```python
from build123d import *

# Parameters (mm, degrees)
SKETCH1_R           = 1.5
BOSS_EXTRUDE1_DEPTH = 5


with BuildPart() as part:
    # Sketch1 → Boss-Extrude1 (new body)
    with BuildSketch(Plane.XY):
        with BuildLine():
            Line((-15, 92), (-10, 97))
            Line((-10, 97), (-5, 97))
            ThreePointArc((-5, 97), (-1.464466094, 98.464466094), (0, 102))
            Line((0, 102), (0, 107))
            ThreePointArc((0, 107), (0.878679656, 109.121320344), (3, 110))
            Line((3, 110), (14.566367929, 110))
            ThreePointArc((14.566367929, 110), (18.101901835, 111.464466094), (19.566367929, 115))
            Line((19.566367929, 115), (19.566367929, 142))
            Line((19.566367929, 142), (22.566367929, 145))
            Line((22.566367929, 145), (86.566367929, 145))
            Line((86.566367929, 145), (89.566367929, 142))
            Line((89.566367929, 142), (89.566367929, 115))
            ThreePointArc((89.566367929, 115), (91.030834023, 111.464466094), (94.566367929, 110))
            Line((94.566367929, 110), (106.132735857, 110))
            ThreePointArc((106.132735857, 110), (108.254056201, 109.121320344), (109.132735857, 107))
            Line((109.132735857, 107), (109.132735857, 102))
            ThreePointArc((109.132735857, 102), (110.597201951, 98.464466094), (114.132735857, 97))
            Line((114.132735857, 97), (119.132735857, 97))
            Line((119.132735857, 97), (124.132735857, 92))
            Line((124.132735857, 92), (124.132735857, 18))
            Line((124.132735857, 18), (119.132735857, 13))
            Line((119.132735857, 13), (114.132735857, 13))
            ThreePointArc((114.132735857, 13), (110.597201951, 11.535533906), (109.132735857, 8))
            Line((109.132735857, 8), (109.132735857, 3))
            ThreePointArc((109.132735857, 3), (108.254056201, 0.878679656), (106.132735857, 0))
            Line((106.132735857, 0), (94.566367929, 0))
            ThreePointArc((94.566367929, 0), (91.030834023, -1.464466094), (89.566367929, -5))
            Line((89.566367929, -5), (89.566367929, -32))
            Line((89.566367929, -32), (86.566367929, -35))
            Line((86.566367929, -35), (22.566367929, -35))
            Line((22.566367929, -35), (19.566367929, -32))
            Line((19.566367929, -32), (19.566367929, -5))
            ThreePointArc((19.566367929, -5), (18.101901835, -1.464466094), (14.566367929, 0))
            Line((14.566367929, 0), (3, 0))
            ThreePointArc((3, 0), (0.878679656, 0.878679656), (0, 3))
            Line((0, 3), (0, 9.1034271))
            ThreePointArc((0, 9.1034271), (-1.464466094, 12.638961006), (-5, 14.1034271))
            Line((-5, 14.1034271), (-10, 14.1034271))
            Line((-10, 14.1034271), (-15, 19.1034271))
            Line((-15, 19.1034271), (-15, 92))
        make_face()
        with Locations((54.566367929, 97)):
            Circle(SKETCH1_R, mode=Mode.SUBTRACT)
        with Locations((54.566367929, 13)):
            Circle(SKETCH1_R, mode=Mode.SUBTRACT)
        with Locations((96.132735857, 55)):
            Circle(SKETCH1_R, mode=Mode.SUBTRACT)
        with Locations((13, 55)):
            Circle(SKETCH1_R, mode=Mode.SUBTRACT)
        with BuildLine():
            Line((34.566367929, 133), (74.566367929, 133))
            ThreePointArc((74.566367929, 133), (76.687688272, 132.121320344), (77.566367929, 130))
            Line((77.566367929, 130), (77.566367929, 118))
            ThreePointArc((77.566367929, 118), (76.687688272, 115.878679656), (74.566367929, 115))
            Line((74.566367929, 115), (34.566367929, 115))
            ThreePointArc((34.566367929, 115), (32.445047585, 115.878679656), (31.566367929, 118))
            Line((31.566367929, 118), (31.566367929, 130))
            ThreePointArc((31.566367929, 130), (32.445047585, 132.121320344), (34.566367929, 133))
        make_face(mode=Mode.SUBTRACT)
        with BuildLine():
            Line((34.566367929, -23), (74.566367929, -23))
            ThreePointArc((74.566367929, -23), (76.687688272, -22.121320344), (77.566367929, -20))
            Line((77.566367929, -20), (77.566367929, -8))
            ThreePointArc((77.566367929, -8), (76.687688272, -5.878679656), (74.566367929, -5))
            Line((74.566367929, -5), (34.566367929, -5))
            ThreePointArc((34.566367929, -5), (32.445047585, -5.878679656), (31.566367929, -8))
            Line((31.566367929, -8), (31.566367929, -20))
            ThreePointArc((31.566367929, -20), (32.445047585, -22.121320344), (34.566367929, -23))
        make_face(mode=Mode.SUBTRACT)
        with BuildLine():
            Line((-7.610040083, 24.1034271), (-7.610040083, 87))
            ThreePointArc((-7.610040083, 87), (-5, 89.610040083), (-2.389959917, 87))
            Line((-2.389959917, 87), (-2.389959917, 24.1034271))
            ThreePointArc((-2.389959917, 24.1034271), (-5, 21.493387017), (-7.610040083, 24.1034271))
        make_face(mode=Mode.SUBTRACT)
        with BuildLine():
            Line((116.74277594, 24.1034271), (116.74277594, 87))
            ThreePointArc((116.74277594, 87), (114.132735857, 89.610040083), (111.522695774, 87))
            Line((111.522695774, 87), (111.522695774, 24.1034271))
            ThreePointArc((111.522695774, 24.1034271), (114.132735857, 21.493387017), (116.74277594, 24.1034271))
        make_face(mode=Mode.SUBTRACT)
        with BuildLine():
            Line((21.529947274, 89.468147489), (88.351003471, 25.308726653))
            ThreePointArc((88.351003471, 25.308726653), (88.386999729, 23.537331865), (86.615604941, 23.501335607))
            Line((86.615604941, 23.501335607), (19.794548743, 87.660756443))
            ThreePointArc((19.794548743, 87.660756443), (19.758552485, 89.432151231), (21.529947274, 89.468147489))
        make_face(mode=Mode.SUBTRACT)
        with BuildLine():
            Line((30.141972391, 90.830211564), (90.687510201, 32.696340879))
            ThreePointArc((90.687510201, 32.696340879), (90.727054178, 30.750360947), (88.781074246, 30.71081697))
            Line((88.781074246, 30.71081697), (28.235536436, 88.844687655))
            ThreePointArc((28.235536436, 88.844687655), (28.195992459, 90.790667587), (30.141972391, 90.830211564))
        make_face(mode=Mode.SUBTRACT)
        with BuildLine():
            Line((39.483266545, 90.686865308), (90.503044374, 41.699321816))
            ThreePointArc((90.503044374, 41.699321816), (90.542042113, 39.780222555), (88.622942851, 39.741224816))
            Line((88.622942851, 39.741224816), (37.603165023, 88.728768307))
            ThreePointArc((37.603165023, 88.728768307), (37.564167284, 90.647867569), (39.483266545, 90.686865308))
        make_face(mode=Mode.SUBTRACT)
        with BuildLine():
            Line((49.153982666, 90.837738164), (90.341625616, 51.290693151))
            ThreePointArc((90.341625616, 51.290693151), (90.381469395, 49.329959822), (88.420736066, 49.290116043))
            Line((88.420736066, 49.290116043), (47.233093116, 88.837161056))
            ThreePointArc((47.233093116, 88.837161056), (47.193249337, 90.797894385), (49.153982666, 90.837738164))
        make_face(mode=Mode.SUBTRACT)
        with BuildLine():
            Line((58.913272098, 90.890808974), (90.212200397, 60.838588511))
            ThreePointArc((90.212200397, 60.838588511), (90.254158107, 58.773827493), (88.189397089, 58.731869782))
            Line((88.189397089, 58.731869782), (56.89046879, 88.784090246))
            ThreePointArc((56.89046879, 88.784090246), (56.84851108, 90.848851264), (58.913272098, 90.890808974))
        make_face(mode=Mode.SUBTRACT)
        with BuildLine():
            Line((68.200844973, 90.997320319), (90.14380499, 69.928398542))
            ThreePointArc((90.14380499, 69.928398542), (90.190005291, 67.654857424), (87.916464173, 67.608657123))
            Line((87.916464173, 67.608657123), (65.973504156, 88.677578901))
            ThreePointArc((65.973504156, 88.677578901), (65.927303856, 90.951120018), (68.200844973, 90.997320319))
        make_face(mode=Mode.SUBTRACT)
        with BuildLine():
            Line((75.985646215, 90.418887754), (89.801777498, 77.153084552))
            ThreePointArc((89.801777498, 77.153084552), (89.839647655, 75.289474178), (87.976037281, 75.251604021))
            Line((87.976037281, 75.251604021), (74.159905999, 88.517407223))
            ThreePointArc((74.159905999, 88.517407223), (74.122035842, 90.381017597), (75.985646215, 90.418887754))
        make_face(mode=Mode.SUBTRACT)
        with BuildLine():
            Line((84.164714184, 90.316514556), (89.552781085, 85.143066673))
            ThreePointArc((89.552781085, 85.143066673), (89.586573484, 83.480124936), (87.923631748, 83.446332537))
            Line((87.923631748, 83.446332537), (82.535564847, 88.619780421))
            ThreePointArc((82.535564847, 88.619780421), (82.501772448, 90.282722157), (84.164714184, 90.316514556))
        make_face(mode=Mode.SUBTRACT)
        with BuildLine():
            Line((20.116699843, 25.040162824), (25.391558074, 19.751335111))
            ThreePointArc((25.391558074, 19.751335111), (27.054841666, 19.749135575), (27.057041202, 21.412419167))
            Line((27.057041202, 21.412419167), (21.782182971, 26.701246879))
            ThreePointArc((21.782182971, 26.701246879), (20.118899379, 26.703446416), (20.116699843, 25.040162824))
        make_face(mode=Mode.SUBTRACT)
        with BuildLine():
            Line((19.858987713, 33.215810662), (33.384828271, 19.654149429))
            ThreePointArc((33.384828271, 19.654149429), (35.248821752, 19.651684473), (35.251286708, 21.515677954))
            Line((35.251286708, 21.515677954), (21.72544615, 35.077339187))
            ThreePointArc((21.72544615, 35.077339187), (19.861452669, 35.079804143), (19.858987713, 33.215810662))
        make_face(mode=Mode.SUBTRACT)
        with BuildLine():
            Line((19.132791007, 40.988220389), (40.614707507, 19.449413025))
            ThreePointArc((40.614707507, 19.449413025), (42.888716002, 19.446405862), (42.891723164, 21.720414358))
            Line((42.891723164, 21.720414358), (21.409806664, 43.259221722))
            ThreePointArc((21.409806664, 43.259221722), (19.135798169, 43.262228884), (19.132791007, 40.988220389))
        make_face(mode=Mode.SUBTRACT)
        with BuildLine():
            Line((19.062870224, 50.276140805), (49.704176763, 19.55368646))
            ThreePointArc((49.704176763, 19.55368646), (51.76936224, 19.550955446), (51.772093254, 21.616140923))
            Line((51.772093254, 21.616140923), (21.130786715, 52.338595268))
            ThreePointArc((21.130786715, 52.338595268), (19.065601238, 52.341326282), (19.062870224, 50.276140805))
        make_face(mode=Mode.SUBTRACT)
        with BuildLine():
            Line((18.930558524, 60.034677598), (59.252807938, 19.6056422))
            ThreePointArc((59.252807938, 19.6056422), (61.21394434, 19.603048781), (61.216537759, 21.564185183))
            Line((61.216537759, 21.564185183), (20.894288344, 61.993220582))
            ThreePointArc((20.894288344, 61.993220582), (18.933151942, 61.995814), (18.930558524, 60.034677598))
        make_face(mode=Mode.SUBTRACT)
        with BuildLine():
            Line((18.897713631, 69.706514762), (68.845514944, 19.626435978))
            ThreePointArc((68.845514944, 19.626435978), (70.76500872, 19.623897628), (70.76754707, 21.543391404))
            Line((70.76754707, 21.543391404), (20.819745757, 71.623470187))
            ThreePointArc((20.819745757, 71.623470187), (18.900251981, 71.626008538), (18.897713631, 69.706514762))
        make_face(mode=Mode.SUBTRACT)
        with BuildLine():
            Line((18.576959915, 79.043400842), (77.850375474, 19.613010658))
            ThreePointArc((77.850375474, 19.613010658), (79.796755446, 19.610436753), (79.79932935, 21.556816725))
            Line((79.79932935, 21.556816725), (20.525913792, 80.98720691))
            ThreePointArc((20.525913792, 80.98720691), (18.57953382, 80.989780815), (18.576959915, 79.043400842))
        make_face(mode=Mode.SUBTRACT)
    extrude(amount=BOSS_EXTRUDE1_DEPTH)


solid = part.part
```
Work out the finished part from the listing and answer in its coordinate system (mm). A direction names the side the tool comes from. Coordinates: 2 decimals unless noted, no trailing zeros. Answer as a JSON object with one key per item and string values.
Q1. Given pin 1 Ø2.5 at (y, z) = (130, 1.5) entering from +X; pin 2 Ø1.5 at (x, z) = (17.5, 2.5) entering from +Y; pin 3 Ø2.5 at (y, z) = (-13.5, 2.5) entering from -X, each flat-ended and moving along its own axis, determine where each tip first touches the part or whether it passes through.
Results list:
{"pin 1": "stops at x = 89.57", "pin 2": "stops at y = 111.62", "pin 3": "stops at x = 19.57"}
Q2. For a pull along X with two mould halves and no side action, classify faces 1 (the cylindrical face through (114.075, 21.494, 2.465)), 2 (the cylindrical face through (90.992, 111.504, 2.465)), 3 (the flat face through (43.52, 45.02, 2.46)), 4 (the flat face through (0, 6, 2)) as pulls with the +X half, pulls with the -X half, needs draft (parallel to the pull), parting line crosses it, or undercut.
Results list:
{"face 1": "undercut", "face 2": "pulls with the +X half", "face 3": "undercut", "face 4": "pulls with the -X half"}
Q3. Which of the six approach directions +Z, -Z, +X, -X, +Y, -Y give full straight-line access (tool end or side, diameter ignored) to faces 5 (the cylindrical face through (-2, 98, 2)), 6 (the flat face through (19.566, -19, 2)), 7 (the flat face through (24.457, 24.02, 2.465))?
Results list:
{"face 5": "+Z, -Z, -X, +Y", "face 6": "+Z, -Z, -X, -Y", "face 7": "+Z, -Z"}
Q4. Consider L1, parallel to Y at x = 13, z = 1.7; L2, parallel to Y at x = 113.5, z = 3.55; L3, parallel to Y at x = 106.5, z = 2.9. Determine where each line is inside the solid, lowest interval first. Write a range as from..to.
Results list:
{"L1": "y = 0..53.5, 56.5..110", "L2": "y = 12.96..21.57, 89.53..97.04", "L3": "y = 0.02..109.98"}
Q5. Find section A-A (z = 4). State how many separate pieces and enclosed holes the cut face has, plus the area to 3 significant figures.
Results list:
{"separate pieces": "1", "enclosed holes": "23", "area": "14,900 mm^2"}
